Read the model definition and answer for the solid it produces. Units are mm, in the model's axes. Give positions to 0.01 mm unless a question says otherwise; leave off trailing zeros. Order: outer loops, then holes, each group sorted by start corner. A loop starts at its lowest first (then second) coordinate and runs counter-clockwise, first axis right, second up.
Item 1: Given pin 1 Ø1.5 at (y, z) = (-1, 72.5) entering from +X; pin 2 Ø4 at (x, z) = (2.5, 75) entering from -Y; pin 3 Ø2 at (x, z) = (3.5, 64) entering from +Y, each flat-ended and moving along its own axis, determine where each tip first touches the part or whether it passes through.
Item 2: Find the intervals of material crossed by line 1 along Y through (x, z) = (0, 49); line 2 along Y through (x, z) = (0.5, 49.5), in increasing order.
Item 3: The mould has two halves that part along Y. Classify faces 1 (the face through (-0.54, -2.44, 49.36)), 2 (the face through (-1.08, -4.88, 49.3)): +Y half, -Y half, draft (parallel to the pull), parting line (faces both ways), or undercut.
Item 4: A cutting plane is placed at C-C (z = 22). Write down the section's boundary in (x, y).
Item 5: A cutting plane is placed at A-A (y = 0). Write down the section's boundary in (x, z).
from build123d import *

# Parameters (mm, degrees)
F0_R     = 5
F0_R_2   = 2.5
F1_DEPTH = 100


# Not quite as in the source:
# - a fillet or chamfer that OpenCascade refuses, or shapes differently, is made with other operations: its cross-section is extruded or revolved along the edge and cut away or added


with BuildPart() as f1:
    # F0 (on Top) → F1 (new body)
    with BuildSketch(Plane.XY):
        Circle(F0_R)
        Circle(F0_R_2, mode=Mode.SUBTRACT)
    extrude(amount=F1_DEPTH)

    # F2: fillet of radius 5 on 1 edges, made by hand

    # F2_s1 → F2_t2 (revolve, cut)
    with BuildSketch(Plane.XZ):
        with BuildLine():
            ThreePointArc((2.5, 95.6698729811), (3.1698729811, 98.1698729811), (5, 100))
            Line((5, 100), (2.5, 100))
            Line((2.5, 100), (2.5, 95.6698729811))
        make_face()
    revolve(axis=Axis((0, 0, 100), (0, 0, 1)), mode=Mode.SUBTRACT)

    # F3: fillet of radius 5 on 1 edges, made by hand

    # F3_s1 → F3_t2 (revolve, cut)
    with BuildSketch(Plane.XZ):
        with BuildLine():
            ThreePointArc((5, 0), (3.1698729811, 1.8301270189), (2.5, 4.3301270189))
            Line((2.5, 4.3301270189), (2.5, 0))
            Line((2.5, 0), (5, 0))
        make_face()
    revolve(axis=Axis((0, 0, 0), (0, 0, 1)), mode=Mode.SUBTRACT)


solid = f1.part
Response values:
1. pin 1: stops at x = 4.99
1. pin 2: stops at y = -4.97
1. pin 3: stops at y = 4.33
2. line 1: y = -5 to -2.5, 2.5 to 5
2. line 2: y = -4.97 to -2.45, 2.45 to 4.97
3. face 1: undercut
3. face 2: parting line
4. outline: circle Ø10 at (0, 0); hole circle Ø5 at (0, 0)
5. outline: (-5, 0) arc R5 ccw to (-2.5, 4.33) - (-2.5, 95.67) arc R5 ccw to (-5, 100) - close; (2.5, 4.33) arc R5 ccw to (5, 0) - (5, 100) arc R5 ccw to (2.5, 95.67) - close
